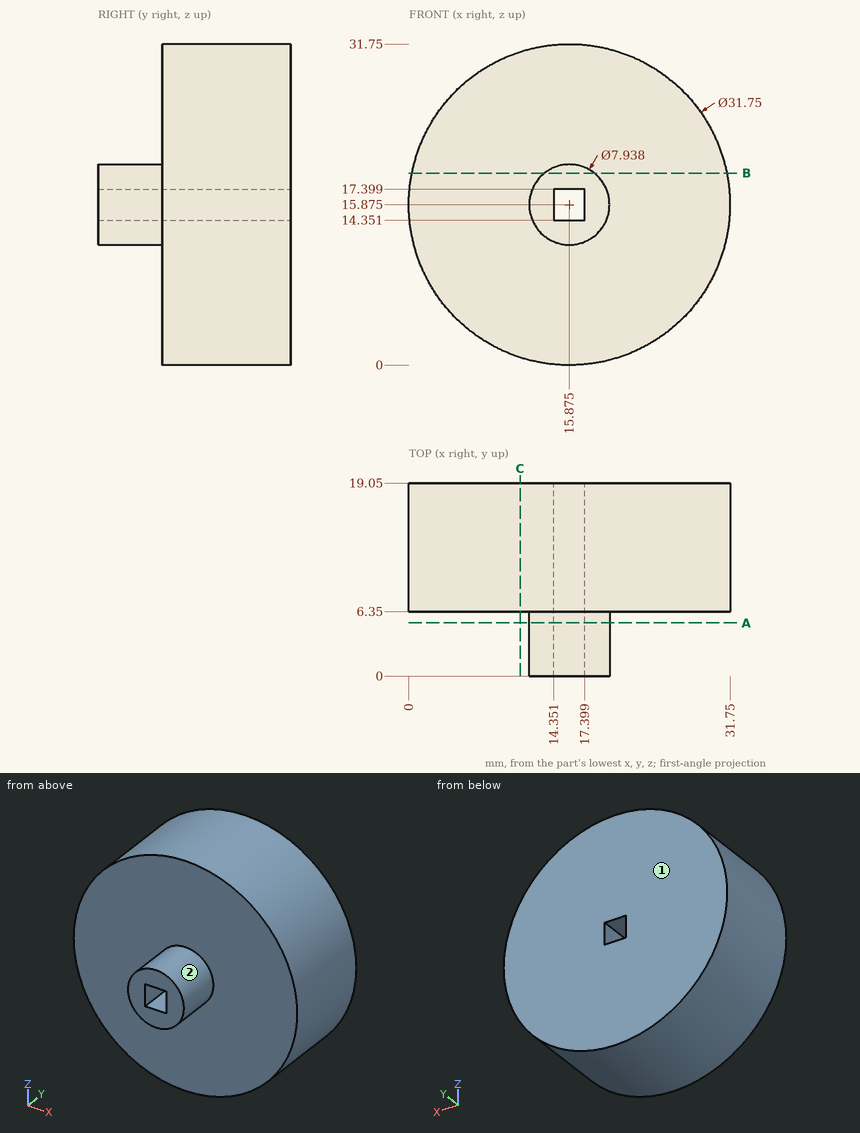
Geometry check sheet. Reference: drawing and pictorial views, mm from the part's lowest x, y, z. A direction names the side the tool comes from. Round coordinates to 2 decimals unless told otherwise and drop trailing zeros. Loops run counter-clockwise (first coordinate to the right, second up) from the corner with the lowest first, then second, coordinate; pieces in that order, holes last. Notation, with made-up numbers: M 1,12.5 L 36,12.5 A20 ccw 36,34.5 Z; hole C 34.25,16 d6. An arc over 180 degrees is marked long. Return JSON: item names as keys, results as strings. Group by question number.
(1) Section check B-B, the plane z = 19. Enter the section's corners in (x, y), and give its area (3 significant figures).
(2) Section check A-A, the plane y = 5.25. Enter the section's corners in (x, z) (1 decimal), and give its area (3 significant figures).
(3) Set-up check for the marked faces 1 and 2: record each of +Z, -Z, +X, -X, +Y, -Y from which the full face is reachable in a straight line by a thin tool's end or side.
(4) Go/stop test with flat-tipped pins: pin 1 (4 mm diameter, centred on y = 5.5, z = 8.5, fed in from +X); pin 2 (1.5 mm diameter, centred on x = 24, y = 8, fed in from +Z); pin 3 (1 mm diameter, centred on y = 8.5, z = 5, fed in from +X). Record where each tip stops, or that it passes through.
(5) Scan lines: line 1 along X through (y, z) = (13.75, 16); line 2 along Y through (x, z) = (20.5, 2); line 3 along Z through (x, y) = (20.5, 6.5). Record each from-to range of solid material in increasing order. Write a range as [from, to].
(6) Section check C-C, the plane x = 11. Enter the section's corners in (y, z).
Data:
{
 "1": {"outline": "M 0.31,6.35 L 13.43,6.35 L 13.43,0 L 18.32,0 L 18.32,6.35 L 31.44,6.35 L 31.44,19.05 L 0.31,19.05 Z", "area": "426 mm²"},
 "2": {"outline": "C 15.9,15.9 d7.9; hole M 14.4,14.4 L 17.4,14.4 L 17.4,17.4 L 14.4,17.4 Z", "area": "40.2 mm²"},
 "3": {"face 1": "+Z, -Z, +X, -X, +Y", "face 2": "-Y"},
 "4": {"pin 1": "x = 30.74", "pin 2": "z = 29.93", "pin 3": "x = 27.89"},
 "5": {"line 1": "[0, 14.35], [17.4, 31.75]", "line 2": "[6.35, 19.05]", "line 3": "[0.69, 31.06]"},
 "6": {"outline": "M 6.35,0.77 L 19.05,0.77 L 19.05,30.98 L 6.35,30.98 Z"}
}
